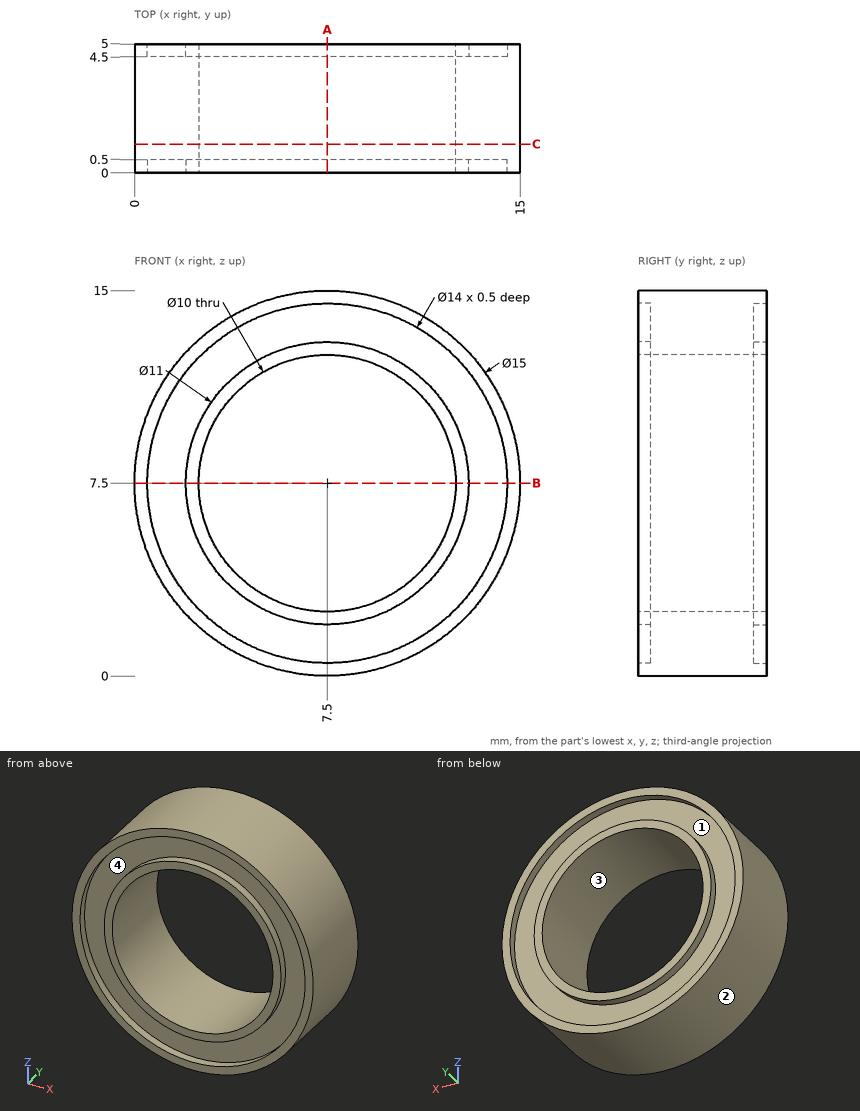
Drawing for the job (mm, zero at the part's lowest x, y, z). A direction names the side the tool comes from. Round coordinates to 2 decimals unless told otherwise and drop trailing zeros. Loops run counter-clockwise (first coordinate to the right, second up) from the corner with the lowest first, then second, coordinate; pieces in that order, holes last. Notation, with made-up numbers: (81.5, -14.75) -> (103.5, -14.75) arc R11 ccw to (103.5, 2.25) -> close; hole circle Ø1 at (-33.5, 84.25). An arc over 180 degrees is marked (long way). Answer in a Markdown table with one row per item.
Item 1: Drill centre lines: L1, parallel to Z at x = 7.5, y = 0.3; L2, parallel to X at y = 0.2, z = 10.5. Where is each one in solid material? Low to high. Write a range as [from, to].
Answers below:
| item | result |
|---|---|
| L1 | z = [0, 0.5], [2, 2.5], [12.5, 13], [14.5, 15] |
| L2 | x = [0.63, 1.18], [2.89, 3.5], [11.5, 12.11], [13.82, 14.37] |
Item 2: Saw through at C-C (y = 1.1). Write the cut outline in (x, z).
Answers below:
| item | result |
|---|---|
| outline | circle Ø15 at (7.5, 7.5); hole circle Ø10 at (7.5, 7.5) |
Item 3: Pin check, flat tips, straight feed: pin 1 (1.5 mm diameter, centred on x = 6, y = 1.5, fed in from +Z); pin 2 (2 mm diameter, centred on y = 4.5, z = 2, fed in from +X); pin 3 (3 mm diameter, centred on x = 11.5, y = 4, fed in from +Z). Stop position of each tip, or through.
Answers below:
| item | result |
|---|---|
| pin 1 | stops at z = 14.96 |
| pin 2 | stops at x = 13.5 |
| pin 3 | stops at z = 14.57 |
Item 4: Saw through at A-A (x = 7.5). Write the cut outline in (y, z).
Answers below:
| item | result |
|---|---|
| outline | (0, 0) -> (5, 0) -> (5, 0.5) -> (4.5, 0.5) -> (4.5, 2) -> (5, 2) -> (5, 2.5) -> (0, 2.5) -> (0, 2) -> (0.5, 2) -> (0.5, 0.5) -> (0, 0.5) -> close; (0, 12.5) -> (5, 12.5) -> (5, 13) -> (4.5, 13) -> (4.5, 14.5) -> (5, 14.5) -> (5, 15) -> (0, 15) -> (0, 14.5) -> (0.5, 14.5) -> (0.5, 13) -> (0, 13) -> close |
Item 5: Which spindle directions (+Z, -Z, +X, -X, +Y, -Y) get a long thin tool onto all of the face, cutting with end or side? Do the marked faces 3 and 4. Say none if no direction does.
Answers below:
| item | result |
|---|---|
| face 3 | +Y, -Y |
| face 4 | -Y |
Item 6: Saw through at B-B (z = 7.5). Write the cut outline in (x, y).
Answers below:
| item | result |
|---|---|
| outline | (0, 0) -> (0.5, 0) -> (0.5, 0.5) -> (2, 0.5) -> (2, 0) -> (2.5, 0) -> (2.5, 5) -> (2, 5) -> (2, 4.5) -> (0.5, 4.5) -> (0.5, 5) -> (0, 5) -> close; (12.5, 0) -> (13, 0) -> (13, 0.5) -> (14.5, 0.5) -> (14.5, 0) -> (15, 0) -> (15, 5) -> (14.5, 5) -> (14.5, 4.5) -> (13, 4.5) -> (13, 5) -> (12.5, 5) -> close |
Item 7: Mould opens along X. For the marked faces 1 and 2 say: +X half, -X half, draft (parallel to the pull), parting line (faces both ways), or undercut.
Answers below:
| item | result |
|---|---|
| face 1 | undercut |
| face 2 | parting line |
